```python
from build123d import *

# Parameters (mm, degrees)
EXTRUDE016_DEPTH = 6
EXTRUDE017_DEPTH = 3
EXTRUDE026_DEPTH = 9
EXTRUDE015_DEPTH = 1
CHAMFER_SIZE     = 2


with BuildPart() as lockbodycutout:
    # Sketch021 → Extrude016 (new body)
    with BuildSketch(Plane.XZ):
        with BuildLine():
            Line((-20, 26), (19, 26))
            ThreePointArc((25, 20), (23.242641, 24.242641), (19, 26))
            Line((25, 20), (25, -18))
            ThreePointArc((19, -24), (23.242641, -22.242641), (25, -18))
            Line((19, -24), (-20, -24))
            Line((-20, -24), (-20, 26))
        make_face()
    extrude(amount=EXTRUDE016_DEPTH)


with BuildPart() as lockbodycutout_1:
    # Extrude016 placement: moved
    add(lockbodycutout.part.moved(Location((150, 7, 0))))


with BuildPart() as lockmountcutout:
    # Sketch024 → Extrude017 (new body)
    with BuildSketch(Plane.XZ):
        with BuildLine():
            Line((-20, 32), (19, 32))
            ThreePointArc((25, 26), (23.242641, 30.242641), (19, 32))
            Line((25, 26), (25, -24))
            ThreePointArc((19, -30), (23.242641, -28.242641), (25, -24))
            Line((19, -30), (-20, -30))
            Line((-20, -30), (-20, 32))
        make_face()
    extrude(amount=EXTRUDE017_DEPTH)


with BuildPart() as lockmountcutout_1:
    # Extrude017 placement: moved
    add(lockmountcutout.part.moved(Location((150, 10, 0))))


with BuildPart() as keyhole:
    # Sketch034 → Extrude026 (new body)
    with BuildSketch(Plane.XZ):
        with BuildLine():
            ThreePointArc((1.5, -2.304886), (0, 2.75), (-1.5, -2.304886))
            Line((-1.5, -2.304886), (-1.5, -8))
            Line((-1.5, -8), (1.5, -8))
            Line((1.5, -8), (1.5, -2.304886))
        make_face()
    extrude(amount=EXTRUDE026_DEPTH)


with BuildPart() as keyhole_1:
    # Extrude026 placement: moved
    add(keyhole.part.moved(Location((150, 1, 0))))


with BuildPart() as doorcutouts:
    # Sketch018 → Extrude015 (new body, symmetric)
    with BuildSketch(Plane.XZ):
        with BuildLine():
            ThreePointArc((157, 3), (150, 10), (143, 3))
            Line((143, 3), (143, -8))
            ThreePointArc((143, -8), (150, -15), (157, -8))
            Line((157, -8), (157, 3))
        make_face()
    extrude(amount=EXTRUDE015_DEPTH, both=True)


with BuildPart() as doorcutouts_1:
    # Extrude015 placement: moved
    add(doorcutouts.part.moved(Location((0, -9, 0))))

    # Fusion: union LockBodyCutout, LockMountCutout, Keyhole
    add(lockbodycutout_1.part)
    add(lockmountcutout_1.part)
    add(keyhole_1.part)


with BuildPart() as door:
    # Sweep001: sweep along a path in Sketch001
    with BuildLine(Plane.XZ) as sweep001_path:
        ThreePointArc((180, 200), (0, 380), (-180, 200))
        Line((-180, 200), (-180, -200))
        ThreePointArc((-180, -200), (0, -380), (180, -200))
        Line((180, -200), (180, 200))
    # Sketch006 → Sweep001 (sweep)
    with BuildSketch(Plane.XY):
        Polygon((120, -10), (120, -5), (130, -5), (130, 10), (180, 10), (180, -10), align=None)
    sweep(path=sweep001_path.line)

    # Cut: cut DoorCutouts
    add(doorcutouts_1.part, mode=Mode.SUBTRACT)

    # Chamfer
    chamfer_edges = [door.edges().sort_by_distance(p)[0] for p in [
        (0, -10, 320),
        (0, -10, 380),
        (120, -10, 0),
        (-120, -10, 0),
        (0, 10, 380),
        (180, -10, 0),
        (-180, -10, 0),
        (0, -10, -320),
        (180, 10, 0),
        (-180, 10, 0),
        (0, -10, -380),
        (0, 10, -380),
    ]]
    chamfer(chamfer_edges, length=CHAMFER_SIZE)


solid = door.part
```
Could you check a few things on this model? Use its own coordinates, in mm. A direction names the side the tool comes from. Coordinates: 2 decimals unless noted, no trailing zeros. Order: outer loops, then holes, each group sorted by start corner. A loop starts at its lowest first (then second) coordinate and runs counter-clockwise, first axis right, second up. Notation, with made-up numbers: M 38.25,-14.75 L 50.25,-14.75 A12 ccw 50.25,-4.75 Z; hole C 23,85.25 d6. An arc over 180 degrees is marked long. Use a Markdown table: item, result. Add a question column.
Q1. I want a section at A-A on x = 0. List the corners of the cut face in (y, z) for me, then the cut area to 3 significant figures.
Q2. I want a section at B-B on z = 178.5. List the corners of the cut face in (x, y) for me.
Q3. Which directions (+Z, -Z, +X, -X, +Y, -Y) give clear straight access to the entire face, cutting with the end or side of a thin tool? Please do faces 1 (the conical face through (3.921, 9.681, 378.276)), 2 (the cylindrical face through (2.64, -6.52, 319.97)), 3 (the cylindrical face through (2.86, 2.39, 329.97)), 4 (the flat face through (-180, 0, -3)), 5 (the flat face through (147, -8, -2)).
Q4. I'm going to push flat-ended pins straight in: pin 1 (2.5 mm diameter, centred on x = 142, y = 8, fed in from +Z); pin 2 (13 mm diameter, centred on x = 157.5, z = 25, fed in from +Y); pin 3 (12 mm diameter, centred on x = 105, y = 3, fed in from +Z). Where does each tip first touch, or does it pass through?
Q5. If I drill on L1, parallel to X at y = -5.5, z = 0; L2, parallel to X at y = -2, z = 0; L3, parallel to X at y = -0.5, z = 93.5, over which ranges is the centre line in solid material (lowest first)?
Q6. We'd pull the mould along X, two halves only. Please class faces 6 (the conical face through (-3.917, -9.875, -378.082)), 7 (the flat face through (-131, 10, -2)), 8 (the flat face through (130, -1, 3)): pulls with the +X half, pulls with the -X half, needs draft (parallel to the pull), parting line crosses it, or undercut.
Checked values:
| question | item | result |
|---|---|---|
| 1 | outline | M -10,-378 L -8,-380 L 8,-380 L 10,-378 L 10,-330 L -5,-330 L -5,-320 L -8,-320 L -10,-322 Z; M -10,322 L -8,320 L -5,320 L -5,330 L 10,330 L 10,378 L 8,380 L -8,380 L -10,378 Z |
| 1 | area | 2,090 mm² |
| 2 | outline | M -180,-8 L -178,-10 L -122,-10 L -120,-8 L -120,-5 L -130,-5 L -130,10 L -178,10 L -180,8 Z; M 120,-8 L 122,-10 L 178,-10 L 180,-8 L 180,8 L 178,10 L 130,10 L 130,-5 L 120,-5 Z |
| 3 | face 1 | +Z, +Y |
| 3 | face 2 | +Y, -Y |
| 3 | face 3 | +Y |
| 3 | face 4 | +Z, -Z, -X, +Y, -Y |
| 3 | face 5 | -Y |
| 4 | pin 1 | z = 312.2 |
| 4 | pin 2 | y = 7 |
| 4 | pin 3 | z = 350.33 |
| 5 | L1 | -180 to -120, 120 to 147.25, 152.75 to 180 |
| 5 | L2 | -180 to -130, 130 to 147.25, 152.75 to 180 |
| 5 | L3 | -180 to -130, 130 to 180 |
| 6 | face 6 | parting line crosses it |
| 6 | face 7 | needs draft |
| 6 | face 8 | undercut |
